Verification items for the finished model (mm, model axes). A direction names the side the tool comes from. Give positions to 0.01 mm unless a question says otherwise; leave off trailing zeros. Loops run counter-clockwise (first coordinate to the right, second up) from the corner with the lowest first, then second, coordinate; pieces in that order, holes last. Notation, with made-up numbers: (14, 68) -> (66, 68) arc R20 cw to (66, 99) -> close; hole circle Ø2 at (63, 65.5). An arc over 180 degrees is marked (long way). Answer in a Markdown table with one row per item. Add a question column.
Q1. Set-up check for faces 1 (the face through (15.821, 6.465, 20.633)), 2 (the face through (-29.276, 2.028, -14.712)), 3 (the face through (-27, 0, -8)): record each of +Z, -Z, +X, -X, +Y, -Y from which the full face is reachable in a straight line by a thin tool's end or side.
Q2. Material ranges on probe 1 along X at (y, z) = (-1.95, 0); probe 2 along Z at (x, y) = (-27, 1.5); probe 3 along X at (y, z) = (7, 0), recorded low to high.
Q3. Release check for a two-part mould opening along X. For faces 4 (the face through (18.5, 4, 18.5)), 5 (the face through (24.397, -2.028, -12.69)), 6 (the face through (0.751, -1.224, 2.385)) record: pulls with the +X half, pulls with the -X half, needs draft (parallel to the pull), parting line crosses it, or undercut.
Q4. Section check D-D on z = 12.5. Enter the section's corners in (x, y).
Q5. Section check A-A on z = 0. Give the number of separate pieces and of enclosed holes in the cut face, and give its area (3 significant figures).
Q6. Section check B-B on x = -14. Enter the section's corners in (y, z), and give its area (3 significant figures).
Q7. Gauge pin test, flat ends, axial feed: P1, Ø5, axis at y = 1.5, z = -18.5, coming from the +X side; P2, Ø5, axis at x = -27.28, z = -15.75, coming from the +Y side; P3, Ø6.5, axis at x = 0, z = -12.5, coming from the +Y side. Record the tip position at first contact, or that the pin passes through.
Q8. Section check C-C on y = 8. Enter the section's corners in (x, z).
```python
from build123d import *

# Parameters (mm, degrees)
SKETCH2_R                   = 2.25
CUT_EXTRUDE1_DEPTH          = 52.536394907
SKETCH4_R                   = 2.5
CUT_EXTRUDE3_DEPTH          = 10
M6_TAPPED_HOLE1_D           = 5
M6_TAPPED_HOLE1_DEPTH       = 15
M6_TAPPED_HOLE1_CSINK_D     = 6.05
M6_TAPPED_HOLE1_CSINK_ANGLE = 90
M6_TAPPED_HOLE1_TIP         = 1.502151548
SKETCH9_R                   = 2.5
CUT_EXTRUDE4_DEPTH          = 52.39066063
M6_TAPPED_HOLE2_D           = 5
M6_TAPPED_HOLE2_DEPTH       = 65
M6_TAPPED_HOLE2_CSINK_D     = 6.05
M6_TAPPED_HOLE2_CSINK_ANGLE = 90
M6_TAPPED_HOLE2_TIP         = 1.502151548


with BuildPart() as part:
    # Sketch1 → Revolve1 (revolve)
    with BuildSketch(Plane.XY, mode=Mode.PRIVATE) as revolve1_sk:
        Polygon((27.5, 0), (27.5, -4), (0, -4), (0, 2), (17.5, 2), (17.5, 9), (26, 9), (26, 4), (36, 4), (36, 0), align=None)
    revolve(revolve1_sk.sketch.rotate(Axis((0, 0, 0), (0, 1, 0)), 90), axis=Axis((0, 0, 0), (0, 1, 0)))

    # Sketch2 → Cut-Extrude1 (cut, through all)
    with BuildSketch(Plane(origin=(0, 4, 0), x_dir=(1, 0, 0), z_dir=(0, 1, 0))):
        with Locations(Location((0, 31.5, 0), (0, 0, 270))):
            Circle(SKETCH2_R)
        with Locations(Location((27.279800219, 15.75, 0), (0, 0, 270))):
            Circle(SKETCH2_R)
        with Locations(Location((27.279800219, -15.75, 0), (0, 0, 270))):
            Circle(SKETCH2_R)
        with Locations(Location((0, -31.5, 0), (0, 0, 270))):
            Circle(SKETCH2_R)
        with Locations(Location((-27.279800219, -15.75, 0), (0, 0, 270))):
            Circle(SKETCH2_R)
        with Locations(Location((-27.279800219, 15.75, 0), (0, 0, 270))):
            Circle(SKETCH2_R)
    extrude(amount=-CUT_EXTRUDE1_DEPTH, mode=Mode.SUBTRACT)

    # Sketch4 → Cut-Extrude3 (cut)
    with BuildSketch(Plane(origin=(0, 2, 0), x_dir=(1, 0, 0), z_dir=(0, 1, 0))):
        with Locations(Location((12.5, 0, 0), (0, 0, 270))):
            Circle(SKETCH4_R)
        with Locations(Location((0, -12.5, 0), (0, 0, 270))):
            Circle(SKETCH4_R)
        with Locations(Location((-12.5, 0, 0), (0, 0, 270))):
            Circle(SKETCH4_R)
        with Locations(Location((0, 12.5, 0), (0, 0, 270))):
            Circle(SKETCH4_R)
    extrude(amount=-CUT_EXTRUDE3_DEPTH, mode=Mode.SUBTRACT)

    # M6 Tapped Hole1
    with Locations(Plane(origin=(-12.5, 9, 0), x_dir=(0, 0, 1), z_dir=(0, 1, 0))):
        with Locations((0, 0), (0, 25), (-12.5, 12.5), (12.5, 12.5)):
            CounterSinkHole(M6_TAPPED_HOLE1_D / 2, M6_TAPPED_HOLE1_CSINK_D / 2, depth=M6_TAPPED_HOLE1_DEPTH, counter_sink_angle=M6_TAPPED_HOLE1_CSINK_ANGLE)
            with Locations((0, 0, -(M6_TAPPED_HOLE1_DEPTH + M6_TAPPED_HOLE1_TIP / 2))):  # 118° drill point
                Cone(0, M6_TAPPED_HOLE1_D / 2, M6_TAPPED_HOLE1_TIP, mode=Mode.SUBTRACT)

    # Sketch9 → Cut-Extrude4 (cut, through all)
    with BuildSketch(Plane(origin=(0, 2, 0), x_dir=(1, 0, 0), z_dir=(0, 1, 0))):
        with Locations(Location((0, 0, 0), (0, 0, 270))):
            Circle(SKETCH9_R)
    extrude(amount=-CUT_EXTRUDE4_DEPTH, mode=Mode.SUBTRACT)

    # M6 Tapped Hole2
    with Locations(Plane.ZX.offset(2)):
        with Locations((0, 0)):
            CounterSinkHole(M6_TAPPED_HOLE2_D / 2, M6_TAPPED_HOLE2_CSINK_D / 2, depth=M6_TAPPED_HOLE2_DEPTH, counter_sink_angle=M6_TAPPED_HOLE2_CSINK_ANGLE)
            with Locations((0, 0, -(M6_TAPPED_HOLE2_DEPTH + M6_TAPPED_HOLE2_TIP / 2))):  # 118° drill point
                Cone(0, M6_TAPPED_HOLE2_D / 2, M6_TAPPED_HOLE2_TIP, mode=Mode.SUBTRACT)


solid = part.part
```
Taken from the geometry:
| question | item | result |
|---|---|---|
| 1 | face 1 | +Y |
| 1 | face 2 | +Y, -Y |
| 1 | face 3 | -Y |
| 2 | probe 1 | x = -27.5 to -15, -10 to -2.5, 2.5 to 10, 15 to 27.5 |
| 2 | probe 2 | z = -23.81 to -17.98, -13.52 to 13.52, 17.98 to 23.81 |
| 2 | probe 3 | x = -26 to -17.5, 17.5 to 26 |
| 3 | face 4 | needs draft |
| 3 | face 5 | parting line crosses it |
| 3 | face 6 | undercut |
| 4 | outline | (-33.76, 0) -> (-24.49, 0) -> (-24.49, -4) -> (-2.5, -4) -> (-2.5, 2) -> (-12.25, 2) -> (-12.25, 9) -> (-22.8, 9) -> (-22.8, 4) -> (-33.76, 4) -> close; (2.5, -4) -> (24.49, -4) -> (24.49, 0) -> (33.76, 0) -> (33.76, 4) -> (22.8, 4) -> (22.8, 9) -> (12.25, 9) -> (12.25, 2) -> (2.5, 2) -> close |
| 5 | separate pieces | 4 |
| 5 | enclosed holes | 0 |
| 5 | area | 433 mm² |
| 6 | outline | (-4, -23.67) -> (0, -23.67) -> (0, -33.17) -> (4, -33.17) -> (4, -21.91) -> (9, -21.91) -> (9, -10.5) -> (2, -10.5) -> (2, -2) -> (-4, -2) -> close; (-4, 2) -> (2, 2) -> (2, 10.5) -> (9, 10.5) -> (9, 21.91) -> (4, 21.91) -> (4, 33.17) -> (0, 33.17) -> (0, 23.67) -> (-4, 23.67) -> close |
| 6 | area | 503 mm² |
| 7 | P1 | stops at x = 32.25 |
| 7 | P2 | stops at y = 4 |
| 7 | P3 | stops at y = 2 |
| 8 | outline | circle Ø52 at (0, 0); hole circle Ø35 at (0, 0) |
